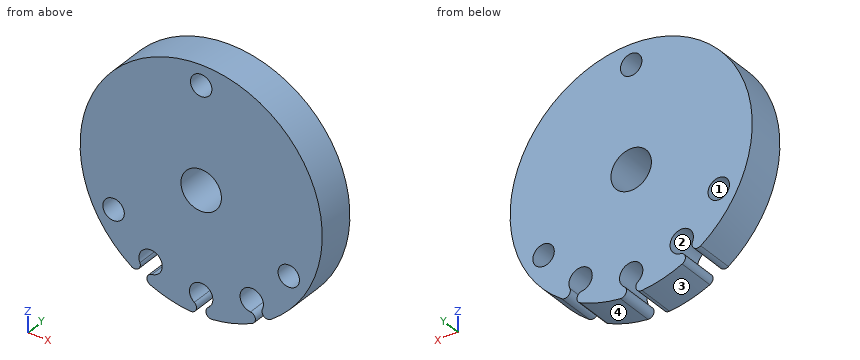
from build123d import *

# Parameters (mm, degrees)
SKETCH1_R           = 19.75
SKETCH1_R_2         = 3.302
SKETCH1_R_3         = 1.75
BOSS_EXTRUDE1_DEPTH = 6.35
CUT_EXTRUDE1_DEPTH  = 7.35
CIRPATTERN1_COUNT   = 3
CIRPATTERN1_ANGLE   = 60


with BuildPart() as part:
    # Sketch1 → Boss-Extrude1 (new body)
    with BuildSketch(Plane(origin=(0, 0, 0), x_dir=(1, 0, 0), z_dir=(0, 1, 0))):
        with Locations(Location((0, 0, 0), (0, 0, 270))):  # turned: the seam where the file's is
            Circle(SKETCH1_R)
        with Locations(Location((0, 0, 0), (0, 0, 270))):  # turned: the seam where the file's is
            Circle(SKETCH1_R_2, mode=Mode.SUBTRACT)
        with Locations(Location((-14.289419162, 8.25, 0), (0, 0, 270))):  # turned: the seam where the file's is
            Circle(SKETCH1_R_3, mode=Mode.SUBTRACT)
        with Locations(Location((0, -16.5, 0), (0, 0, 270))):  # turned: the seam where the file's is
            Circle(SKETCH1_R_3, mode=Mode.SUBTRACT)
        with Locations(Location((14.289419162, 8.25, 0), (0, 0, 270))):  # turned: the seam where the file's is
            Circle(SKETCH1_R_3, mode=Mode.SUBTRACT)
    extrude(amount=BOSS_EXTRUDE1_DEPTH)

    # Sketch2 → Cut-Extrude1 (cut, through all)
    with BuildSketch(Plane(origin=(0, 6.35, 0), x_dir=(1, 0, 0), z_dir=(0, 1, 0))):
        with BuildLine():
            ThreePointArc((8.036161973, 16.182379357), (7.2975, 12.639640768), (9.99627063, 15.050710096))
            ThreePointArc((9.99627063, 15.050710096), (10.255103275, 16.120005739), (11.354562521, 16.159715652))
            ThreePointArc((11.354562521, 16.159715652), (9.875, 17.104001725), (8.317443012, 17.913197418))
            ThreePointArc((8.317443012, 17.913197418), (8.832782842, 16.941182824), (8.036161973, 16.182379357))
        make_face()
    cut_extrude1 = extrude(amount=-CUT_EXTRUDE1_DEPTH, mode=Mode.SUBTRACT)

    # CirPattern1: Cut-Extrude1 ×3 about axis
    cirpattern1_axis = Axis((0, 0, 0), (0, 1, 0))
    for i in range(1, CIRPATTERN1_COUNT):
        add(cut_extrude1.rotate(cirpattern1_axis, i * CIRPATTERN1_ANGLE / (CIRPATTERN1_COUNT - 1)), mode=Mode.SUBTRACT)


solid = part.part
Verification items for the finished model (mm, model axes). Face numbers are marked on the shaded views. Coordinates: 2 decimals unless noted, no trailing zeros. Write each loop counter-clockwise with the first axis right and the second up, starting at its lowest first coordinate (ties: lowest second). Pieces come first, ordered by that corner, then holes. Notation, with made-up numbers: (83, -18) - (94, -18) arc R24 cw to (94, 11) - close; hole circle Ø11 at (15.25, -13.5). An arc over 180 degrees is marked (long way). Answer as a JSON object with one key per item and string values.
(1) Thickness scan on line 1 along X through (y, z) = (1.5, 0); line 2 along X through (y, z) = (2, -8.25); line 3 along X through (y, z) = (0.75, -13.5). Record the ranges inside material, lowest first.
Report:
{"line 1": "-19.75 to -3.3, 3.3 to 19.75", "line 2": "-17.94 to -16.04, -12.54 to 12.54, 16.04 to 17.94", "line 3": "-14.42 to -9.98, -6.52 to 6.52, 9.98 to 14.42"}
(2) Cross-section at D-D on z = -8.25. Record the cut outline in (x, y), plus the area to 3 significant figures.
Report:
{"outline": "(-17.94, 0) - (-16.04, 0) - (-16.04, 6.35) - (-17.94, 6.35) - close; (-12.54, 0) - (12.54, 0) - (12.54, 6.35) - (-12.54, 6.35) - close; (16.04, 0) - (17.94, 0) - (17.94, 6.35) - (16.04, 6.35) - close", "area": "183 mm^2"}
(3) Cross-section at C-C on y = 2. Record the cut outline in (x, z) (3 decimals).
Report:
{"outline": "(-11.355, -16.16) arc R0.911 ccw to (-9.996, -15.051) arc R1.905 cw (long way) to (-8.036, -16.182) arc R0.911 ccw to (-8.317, -17.913) arc R19.75 ccw to (-1.753, -19.672) arc R0.911 ccw to (-1.132, -18.032) arc R1.905 cw (long way) to (1.132, -18.032) arc R0.911 ccw to (1.753, -19.672) arc R19.75 ccw to (8.317, -17.913) arc R0.911 ccw to (8.036, -16.182) arc R1.905 cw (long way) to (9.996, -15.051) arc R0.911 ccw to (11.355, -16.16) arc R19.75 ccw (long way) to start; hole circle Ø3.5 at (-14.289, -8.25); hole circle Ø6.604 at (0, 0); hole circle Ø3.5 at (0, 16.5); hole circle Ø3.5 at (14.289, -8.25)"}
(4) Mould release check, pull along X, two halves, no side actions. Record for the marked faces 1, 2, 3 and 4: pulls with the +X half, pulls with the -X half, needs draft (parallel to the pull), parting line crosses it, or undercut.
Report:
{"face 1": "undercut", "face 2": "undercut", "face 3": "pulls with the -X half", "face 4": "pulls with the +X half"}
(5) Cross-section at B-B on z = 0. Record the cut outline in (x, y).
Report:
{"outline": "(-19.75, 0) - (-3.3, 0) - (-3.3, 6.35) - (-19.75, 6.35) - close; (3.3, 0) - (19.75, 0) - (19.75, 6.35) - (3.3, 6.35) - close"}
(6) Gauge pin test, flat ends, axial feed: pin 1 Ø3.5 at (x, z) = (-8.25, -14.29) entering from +Y; pin 2 Ø2 at (y, z) = (5, -9) entering from -X; pin 3 Ø2 at (x, y) = (-9, 5) entering from +Z. Record the tip position at first contact, or that the pin passes through.
Report:
{"pin 1": "through", "pin 2": "x = -18.06", "pin 3": "z = 18.06"}
(7) Cross-section at A-A on x = 0. Record the cut outline in (y, z) (3 decimals), plus the area to 3 significant figures.
Report:
{"outline": "(0, -14.595) - (6.35, -14.595) - (6.35, -3.302) - (0, -3.302) - close; (0, 3.302) - (6.35, 3.302) - (6.35, 14.75) - (0, 14.75) - close; (0, 18.25) - (6.35, 18.25) - (6.35, 19.75) - (0, 19.75) - close", "area": "154 mm^2"}
